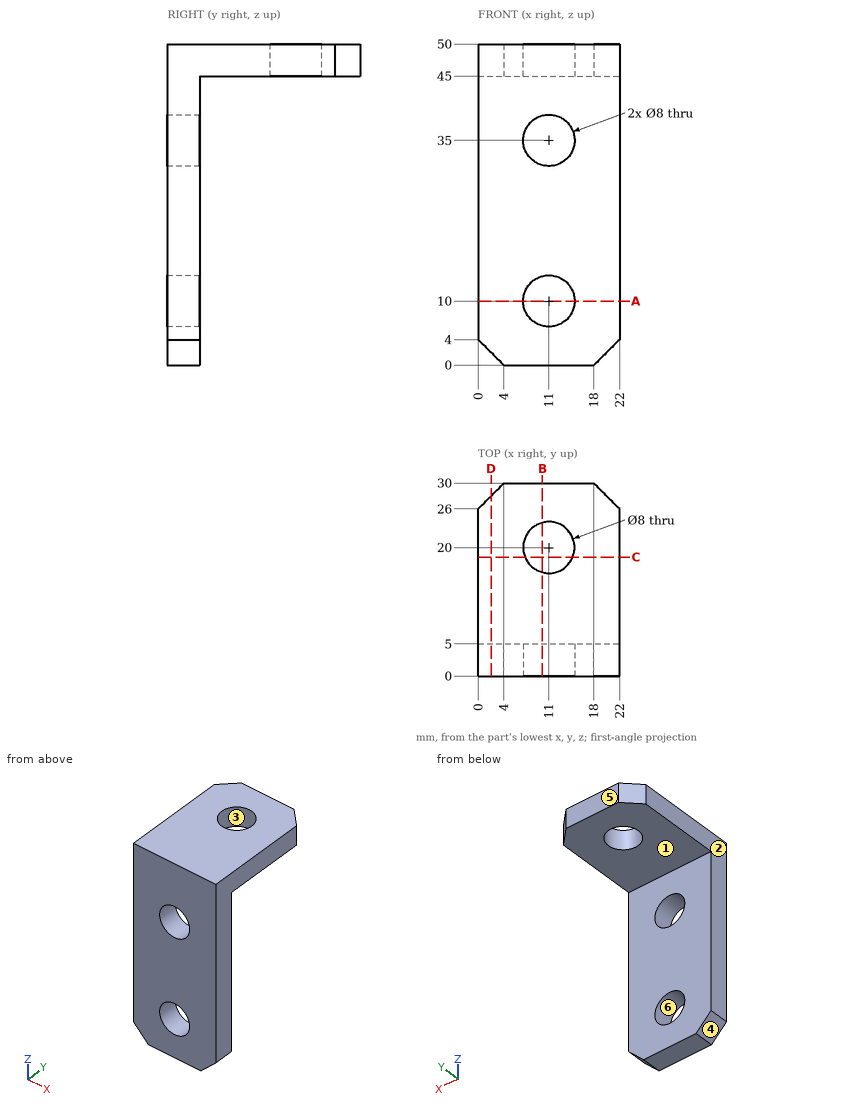
For this review, use the dimensioned drawing (mm, ordinates from the lowest corner) and the shaded views. A direction names the side the tool comes from. Coordinates: 2 decimals unless noted, no trailing zeros. Loops run counter-clockwise (first coordinate to the right, second up) from the corner with the lowest first, then second, coordinate; pieces in that order, holes last. Notation, with made-up numbers: (32, -36.5) -> (67, -36.5) arc R18 cw to (67, -21.5) -> close; hole circle Ø4 at (-37.5, -12.5). An arc over 180 degrees is marked (long way). Return JSON: item names as keys, results as strings. Group by question number.
(1) Consider section C-C, the plane y = 18.5. Give the boundary of the cut face in (x, z), plus the area to 3 significant figures.
(2) Consider section A-A, the plane z = 10. Give the boundary of the cut face in (x, y), plus the area to 3 significant figures.
(3) To check wall thickness, follow L1, parallel to X at y = 1.45, z = 35; L2, parallel to Y at x = 11, z = 46.6; L3, parallel to Z at x = 13.5, y = 3.75. State the ranges of each line that lie inside material, in increasing order.
(4) Mouldability with a two-part tool opening along X and no side actions: class the marked faces 3, 4, 5 and 6 as pulls with the +X half, pulls with the -X half, needs draft (parallel to the pull), parting line crosses it, or undercut.
(5) Consider section D-D, the plane x = 2. Give the boundary of the cut face in (y, z).
(6) Consider section B-B, the plane x = 10. Give the boundary of the cut face in (y, z).
(7) Tool access review of the marked faces 1 and 2: name each direction out of +Z, -Z, +X, -X, +Y, -Y from which nothing blocks a thin tool from reaching the whole face with its end or side.
(8) For pin 1 Ø8 at (x, z) = (17.5, 19.5) entering from +Y; pin 2 Ø6.5 at (x, y) = (13.5, 21) entering from -Z, all flat-tipped, find the tip position at first contact; note any pin that passes through.
Results below:
{
 "1": {"outline": "(0, 45) -> (7.29, 45) -> (7.29, 50) -> (0, 50) -> close; (14.71, 45) -> (22, 45) -> (22, 50) -> (14.71, 50) -> close", "area": "72.9 mm2"},
 "2": {"outline": "(0, 0) -> (7, 0) -> (7, 5) -> (0, 5) -> close; (15, 0) -> (22, 0) -> (22, 5) -> (15, 5) -> close", "area": "70.0 mm2"},
 "3": {"L1": "x = 0 to 7, 15 to 22", "L2": "y = 0 to 16, 24 to 30", "L3": "z = 0 to 6.88, 13.12 to 31.88, 38.12 to 50"},
 "4": {"face 3": "undercut", "face 4": "pulls with the -X half", "face 5": "needs draft", "face 6": "undercut"},
 "5": {"outline": "(0, 2) -> (5, 2) -> (5, 45) -> (28, 45) -> (28, 50) -> (0, 50) -> close"},
 "6": {"outline": "(0, 0) -> (5, 0) -> (5, 6.13) -> (0, 6.13) -> close; (0, 13.87) -> (5, 13.87) -> (5, 31.13) -> (0, 31.13) -> close; (0, 38.87) -> (5, 38.87) -> (5, 45) -> (16.13, 45) -> (16.13, 50) -> (0, 50) -> close; (23.87, 45) -> (30, 45) -> (30, 50) -> (23.87, 50) -> close"},
 "7": {"face 1": "-Z, +X, -X, +Y", "face 2": "+Z, -Z, -X, +Y, -Y"},
 "8": {"pin 1": "stops at y = 5", "pin 2": "stops at z = 45"}
}
